from build123d import *

# Parameters (mm, degrees)
P_IDAT_VYSUNUT_M1_DEPTH  = 4
SKICA2_W                 = 20
SKICA2_H                 = 4
P_IDAT_VYSUNUT_M2_DEPTH  = 15
SKICA3_W                 = 5.5
SKICA3_H                 = 3
ODEBRAT_VYSUNUT_M1_DEPTH = 15
SKICA4_W                 = 20
SKICA4_H                 = 15
ODEBRAT_VYSUNUT_M2_DEPTH = 15
SKICA5_W                 = 4
SKICA5_H                 = 4
P_IDAT_VYSUNUT_M3_DEPTH  = 20
SKICA6_W                 = 1
SKICA6_H                 = 5
ODEBRAT_VYSUNUT_M3_DEPTH = 10


with BuildPart() as part:
    # Skica1 → Přidat vysunutím1 (new body)
    with BuildSketch(Plane.XY):
        Polygon((0, 0), (5, 0), (5, -2), (10, -2), (10, 4.082474227), (10, 13), (30, 13), (30, -2), (35, -2), (35, 18), (5, 18), (5, 5), (0, 5), align=None)
    extrude(amount=P_IDAT_VYSUNUT_M1_DEPTH)

    # Skica2 → Přidat vysunutím2 (add)
    with BuildSketch(Plane(origin=(0, 18, 0), x_dir=(1, 0, 0), z_dir=(0, 1, 0))):
        with Locations((20, -2)):
            Rectangle(SKICA2_W, SKICA2_H)
    extrude(amount=P_IDAT_VYSUNUT_M2_DEPTH)

    # Skica3 → Odebrat vysunutím1 (cut)
    with BuildSketch(Plane.XY.offset(4)):
        with Locations((20, 28)):
            Rectangle(SKICA3_W, SKICA3_H)
    extrude(amount=-ODEBRAT_VYSUNUT_M1_DEPTH, mode=Mode.SUBTRACT)

    # Skica4 → Odebrat vysunutím2 (cut)
    with BuildSketch(Plane.XY.offset(4)):
        with Locations((20, 25.5)):
            Rectangle(SKICA4_W, SKICA4_H)
    extrude(amount=-ODEBRAT_VYSUNUT_M2_DEPTH, mode=Mode.SUBTRACT)

    # Skica5 → Přidat vysunutím3 (add)
    with BuildSketch(Plane(origin=(0, 18, 0), x_dir=(1, 0, 0), z_dir=(0, 1, 0))):
        with Locations((7, -2)):
            Rectangle(SKICA5_W, SKICA5_H)
        with Locations((33, -2)):
            Rectangle(SKICA5_W, SKICA5_H)
    extrude(amount=P_IDAT_VYSUNUT_M3_DEPTH)

    # Skica6 → Odebrat vysunutím3 (cut)
    with BuildSketch(Plane.XY.offset(4)):
        with Locations((0.5, 2.5)):
            Rectangle(SKICA6_W, SKICA6_H)
    extrude(amount=-ODEBRAT_VYSUNUT_M3_DEPTH, mode=Mode.SUBTRACT)


solid = part.part
The model under review builds one solid part; all positions refer to its coordinate system, in mm. A direction names the side the tool comes from. Give positions to 0.01 mm unless a question says otherwise; leave off trailing zeros. Order: outer loops, then holes, each group sorted by start corner. A loop starts at its lowest first (then second) coordinate and runs counter-clockwise, first axis right, second up. Notation, with made-up numbers: M 11,37.5 L 15,37.5 A5 cw 15,46.5 Z; hole C 79.25,-2.5 d1. An arc over 180 degrees is marked long. One line per question, with ' | ' between items. Start each with the question number.
1) Wall thickness on L1, parallel to X at y = 29.5, z = 0.75; L2, parallel to X at y = 0.5, z = 1.2; L3, parallel to Y at x = 10.5, z = 3.15: over which ranges is each line inside the solid? List them lowest first. Write a range as from..to.
2) Mouldability with a two-part tool opening along Z and no side actions: class faces 6 (the face through (17.8, 17.7, 0)), 7 (the face through (17.8, 17.7, 4)), 8 (the face through (31, 28, 2)) as pulls with the +Z half, pulls with the -Z half, needs draft (parallel to the pull), parting line crosses it, or undercut.
3) For faces 1 (the face through (5, -1, 2)), 2 (the face through (5, 21, 2)), 3 (the face through (35, 18, 2)), 4 (the face through (9, 28, 2)), 5 (the face through (20, 13, 2)), list the 3-axis set-ups (+Z, -Z, +X, -X, +Y, -Y) from which the entire face can be reached by the end or side of a thin tool; tool diameter is ignored.
4) Consider section C-C, the plane y = 27. Give the boundary of the cut face in (x, z), then the cut area to 3 significant figures.
5) Consider section A-A, the plane y = 12.5. Give the boundary of the cut face in (x, z).
6) Consider section D-D, the plane y = 16.5. Give the boundary of the cut face in (x, z), then the cut area to 3 significant figures.
7) Clearance check with flat-ended pins moving along their axes: P1, Ø0.6, axis at y = -0.5, z = 1, coming from the -X side; P2, Ø2, axis at x = 17, z = 2, coming from the -Y side. State where each tip first meets the part, or that it passes through.
8) Consider section B-B, the plane z = 1.75. Give the boundary of the cut face in (x, y).
Found:
1) L1: x = 5..9, 31..35 | L2: x = 1..10, 30..35 | L3: y = 13..18
2) face 6: pulls with the -Z half | face 7: pulls with the +Z half | face 8: needs draft
3) face 1: +Z, -Z, -X, -Y | face 2: +Z, -Z, -X, +Y | face 3: +Z, -Z, +X, +Y, -Y | face 4: +Z, -Z, +Y | face 5: +Z, -Z, -Y
4) outline: M 5,0 L 9,0 L 9,4 L 5,4 Z; M 31,0 L 35,0 L 35,4 L 31,4 Z | area: 32.0 mm²
5) outline: M 5,0 L 10,0 L 10,4 L 5,4 Z; M 30,0 L 35,0 L 35,4 L 30,4 Z
6) outline: M 5,0 L 35,0 L 35,4 L 5,4 Z | area: 120 mm²
7) P1: stops at x = 5 | P2: stops at y = 13
8) outline: M 1,0 L 5,0 L 5,-2 L 10,-2 L 10,13 L 30,13 L 30,-2 L 35,-2 L 35,38 L 31,38 L 31,18 L 9,18 L 9,38 L 5,38 L 5,5 L 1,5 Z
